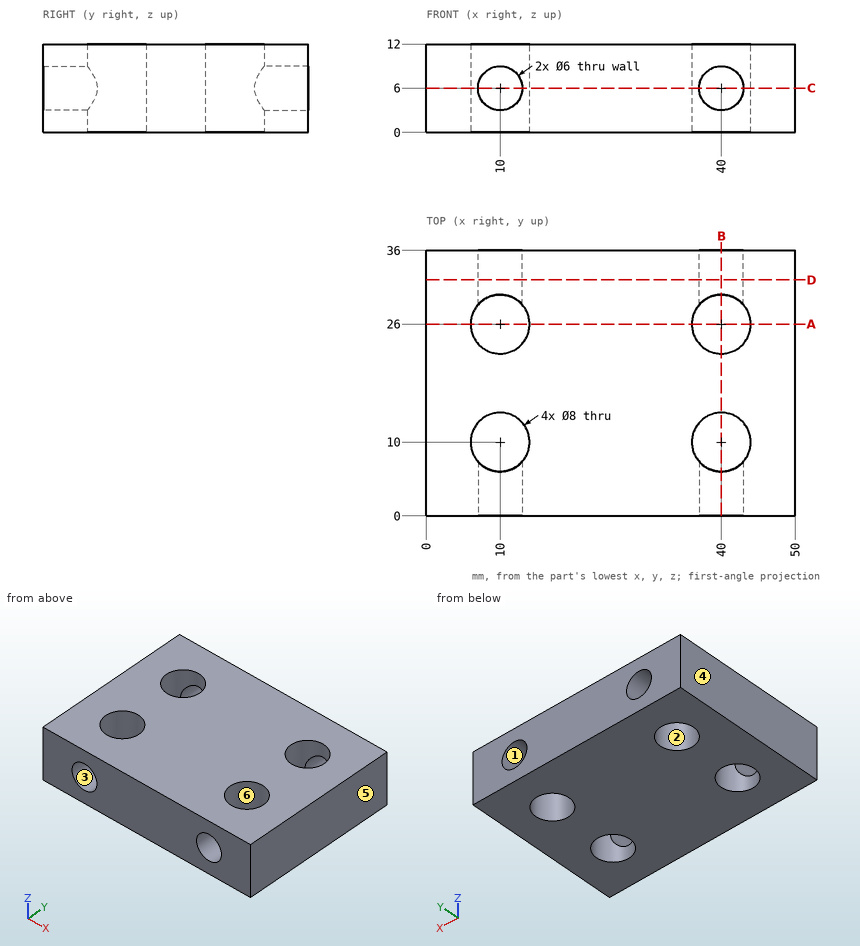
The figure shows three views and two pictorial views of one solid part (mm, origin at its lowest corner). Answer the questions. A direction names the side the tool comes from. Give positions to 0.01 mm unless a question says otherwise; leave off trailing zeros. Loops run counter-clockwise (first coordinate to the right, second up) from the corner with the lowest first, then second, coordinate; pieces in that order, holes last. Notation, with made-up numbers: (57, 53.5) -> (90, 53.5) arc R26 ccw to (90, 87.5) -> close; hole circle Ø11 at (29.25, 14.5). An arc over 180 degrees is marked (long way). Use a Markdown table: item, result. Add a question column.
1. Find the intervals of material crossed by probe 1 along X at (y, z) = (2.25, 6); probe 2 along Z at (x, y) = (10, 33.75); probe 3 along Y at (x, z) = (40, 0.5), in increasing order.
2. Determine the mould class of the marked faces 4, 5 and 6 for opening direction X: released by +X, released by -X, zero draft, split by the parting line, or undercut.
3. Section D-D on y = 32 is taken. Determine the outline of the cut face in (x, z).
4. For the marked faces 1, 2 and 3, determine the directions among +Z, -Z, +X, -X, +Y, -Y from which every point of the face is accessible in a straight line to the end or side of a thin tool.
5. Section C-C on z = 6 is taken. Determine the outline of the cut face in (x, y), and give its area (3 significant figures).
6. Flat-ended cylindrical pins translate along their axes: pin 1 Ø7 at (x, z) = (40, 6) entering from -Y; pin 2 Ø5 at (x, z) = (10, 6) entering from +Y; pin 3 Ø7 at (x, y) = (10, 26) entering from +Z. Find the tip coordinate at first contact, or state that the pin passes through.
7. Section B-B on x = 40 is taken. Determine the outline of the cut face in (y, z).
8. Section A-A on y = 26 is taken. Determine the outline of the cut face in (x, z), and give its area (3 significant figures).
Results below:
| question | item | result |
|---|---|---|
| 1 | probe 1 | x = 0 to 7, 13 to 37, 43 to 50 |
| 1 | probe 2 | z = 0 to 3, 9 to 12 |
| 1 | probe 3 | y = 0 to 6, 14 to 22, 30 to 36 |
| 2 | face 4 | released by -X |
| 2 | face 5 | released by +X |
| 2 | face 6 | undercut |
| 3 | outline | (0, 0) -> (50, 0) -> (50, 12) -> (0, 12) -> close; hole circle Ø6 at (10, 6); hole circle Ø6 at (40, 6) |
| 4 | face 1 | +Y |
| 4 | face 2 | +Z, -Z |
| 4 | face 3 | -Y |
| 5 | outline | (0, 0) -> (7, 0) -> (7, 7.35) arc R4 cw (long way) to (13, 7.35) -> (13, 0) -> (37, 0) -> (37, 7.35) arc R4 cw (long way) to (43, 7.35) -> (43, 0) -> (50, 0) -> (50, 36) -> (43, 36) -> (43, 28.65) arc R4 cw (long way) to (37, 28.65) -> (37, 36) -> (13, 36) -> (13, 28.65) arc R4 cw (long way) to (7, 28.65) -> (7, 36) -> (0, 36) -> close |
| 5 | area | 1,440 mm^2 |
| 6 | pin 1 | stops at y = 0 |
| 6 | pin 2 | stops at y = 22.88 |
| 6 | pin 3 | passes through |
| 7 | outline | (0, 0) -> (6, 0) -> (6, 3) -> (0, 3) -> close; (0, 9) -> (6, 9) -> (6, 12) -> (0, 12) -> close; (14, 0) -> (22, 0) -> (22, 12) -> (14, 12) -> close; (30, 0) -> (36, 0) -> (36, 3) -> (30, 3) -> close; (30, 9) -> (36, 9) -> (36, 12) -> (30, 12) -> close |
| 8 | outline | (0, 0) -> (6, 0) -> (6, 12) -> (0, 12) -> close; (14, 0) -> (36, 0) -> (36, 12) -> (14, 12) -> close; (44, 0) -> (50, 0) -> (50, 12) -> (44, 12) -> close |
| 8 | area | 408 mm^2 |
